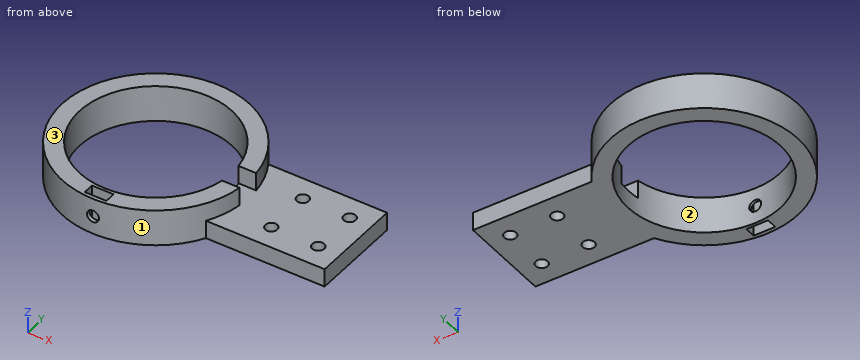
from build123d import *

# Parameters (mm, degrees)
SKETCH1_R              = 51.5
BOSS_EXTRUDE1_DEPTH    = 20
BOSS_EXTRUDE2_DEPTH    = 10
SKETCH2_R              = 41.9
CUT_EXTRUDE1_DEPTH     = 124.094475912
SKETCH3_W              = 35
SKETCH3_H              = 13.351317372
CUT_EXTRUDE2_DEPTH     = 10
SKETCH4_W              = 11.9
SKETCH4_H              = 5.94
CUT_EXTRUDE3_DEPTH     = 124.094475912
CUT_EXTRUDE4_START     = -51.500000101
CUT_EXTRUDE4_OUTLINE_R = 3.3
CUT_EXTRUDE4_DEPTH     = 9.730154575
SKETCH5_R              = 3.3
CUT_EXTRUDE5_DEPTH     = 122.869807632


# Read off the part's stored shape, not the designer's step: Cut-Extrude4
with BuildPart() as part:
    # Sketch1 → Boss-Extrude1 (new body)
    with BuildSketch(Plane.XY):
        Circle(SKETCH1_R)
    extrude(amount=BOSS_EXTRUDE1_DEPTH)

    # 3DSketch1 → Boss-Extrude2 (add)
    with BuildSketch(Plane(origin=(0, -25.55, 0), x_dir=(0.9069189732091603, 0.4213050866453462, 0), z_dir=(0, 0, -1))):
        Polygon((0, 0), (99.761087053, 46.343559531), (121.289776981, 0), (21.528689928, -46.343559531), align=None)
    extrude(amount=-BOSS_EXTRUDE2_DEPTH)

    # Sketch2 → Cut-Extrude1 (cut, through all)
    with BuildSketch(Plane.XY.offset(20)):
        Circle(SKETCH2_R)
    extrude(amount=-CUT_EXTRUDE1_DEPTH, mode=Mode.SUBTRACT)

    # Sketch3 → Cut-Extrude2 (cut)
    with BuildSketch(Plane.XY.offset(20)):
        with Locations((56.5, -0.55960538)):
            Rectangle(SKETCH3_W, SKETCH3_H)
    extrude(amount=-CUT_EXTRUDE2_DEPTH, mode=Mode.SUBTRACT)

    # Sketch4 → Cut-Extrude3 (cut, through all)
    with BuildSketch(Plane.XY.offset(20)):
        with Locations((0, -46.37)):
            Rectangle(SKETCH4_W, SKETCH4_H)
    extrude(amount=-CUT_EXTRUDE3_DEPTH, mode=Mode.SUBTRACT)

    # Cut-Extrude4 outline → Cut-Extrude4 (cut)
    with BuildSketch(Plane(origin=(0, 0, 0), x_dir=(1, 0, 0), z_dir=(0, 1, 0)).offset(CUT_EXTRUDE4_START)):
        with Locations((0, -10)):
            Circle(CUT_EXTRUDE4_OUTLINE_R)
    extrude(amount=CUT_EXTRUDE4_DEPTH, mode=Mode.SUBTRACT)

    # Sketch5 → Cut-Extrude5 (cut, through all)
    with BuildSketch(Plane.XY.offset(10)):
        with Locations((72.2, 12.9)):
            Circle(SKETCH5_R)
        with Locations((98, 12.9)):
            Circle(SKETCH5_R)
        with Locations((98, -12.9)):
            Circle(SKETCH5_R)
        with Locations((72.2, -12.9)):
            Circle(SKETCH5_R)
    extrude(amount=-CUT_EXTRUDE5_DEPTH, mode=Mode.SUBTRACT)


solid = part.part
Input: part model. Units: mm. Frame: model coordinates. Face numbers are marked on the shaded views. Coordinates: 2 decimals unless noted, no trailing zeros. Loops run counter-clockwise (first coordinate to the right, second up) from the corner with the lowest first, then second, coordinate; pieces in that order, holes last.
Q1. Cut plane D-D (y = 12.9). Output: boundary loops of the cut face in (x, z).
Q2. Cut plane C-C (x = 0). Output: boundary loops of the cut face in (y, z), then the cut area to 3 significant figures.
Q3. Draft query along Y for the marked faces 1, 2 and 3. Return one class per face: +Y half, -Y half, draft (parallel to the pull), parting line (faces both ways), or undercut.
Q4. Material intervals for line 1 (Y direction, x = 91, z = 3.5); line 2 (Z direction, x = 0, y = -49.75); line 3 (Y direction, x = 0, z = 12.25), sorted ascending.
Q5. Cut plane A-A (y = 0). Output: boundary loops of the cut face in (x, z).
Q6. Cut plane B-B (x = 98). Output: boundary loops of the cut face in (y, z).
Q7. Contact query for flat-ended pins moving along their axis: pin 1 (12 mm diameter, centred on x = 20.5, z = 4.5, fed in from -Y); pin 2 (1 mm diameter, centred on x = -16.5, z = 15.5, fed in from +Y); pin 3 (5 mm diameter, centred on x = 44, z = 13, fed in from -Y). Output: stop coordinate, or through.
Working result:
1. outline: (-49.86, 0) - (-39.86, 0) - (-39.86, 20) - (-49.86, 20) - close; (39.86, 0) - (68.9, 0) - (68.9, 10) - (49.86, 10) - (49.86, 20) - (39.86, 20) - close; (75.5, 0) - (94.7, 0) - (94.7, 10) - (75.5, 10) - close; (101.3, 0) - (110, 0) - (110, 10) - (101.3, 10) - close
2. outline: (-51.5, 0) - (-49.34, 0) - (-49.34, 6.7) - (-51.5, 6.7) - close; (-51.5, 13.3) - (-49.34, 13.3) - (-49.34, 20) - (-51.5, 20) - close; (-43.4, 0) - (-41.9, 0) - (-41.9, 6.7) - (-43.4, 6.7) - close; (-43.4, 13.3) - (-41.9, 13.3) - (-41.9, 20) - (-43.4, 20) - close; (41.9, 0) - (51.5, 0) - (51.5, 20) - (41.9, 20) - close
2. area: 241 mm2
3. face 1: parting line
3. face 2: undercut
3. face 3: draft
4. line 1: y = -25.55 to 25.55
4. line 2: z = 0 to 6.7, 13.3 to 20
4. line 3: y = 41.9 to 51.5
5. outline: (-51.5, 0) - (-41.9, 0) - (-41.9, 20) - (-51.5, 20) - close; (41.9, 0) - (110, 0) - (110, 10) - (41.9, 10) - close
6. outline: (-25.55, 0) - (-16.2, 0) - (-16.2, 10) - (-25.55, 10) - close; (-9.6, 0) - (9.6, 0) - (9.6, 10) - (-9.6, 10) - close; (16.2, 0) - (25.55, 0) - (25.55, 10) - (16.2, 10) - close
7. pin 1: stops at y = -49.42
7. pin 2: stops at y = 48.95
7. pin 3: stops at y = -30.5
